Design review of the part built by this model. Coordinates are the model's own, in mm. A direction names the side the tool comes from. Give positions to 0.01 mm unless a question says otherwise; leave off trailing zeros. Order: outer loops, then holes, each group sorted by start corner. A loop starts at its lowest first (then second) coordinate and runs counter-clockwise, first axis right, second up. Notation, with made-up numbers: (3, -14) -> (7, -14) arc R19 cw to (7, -3) -> close; hole circle Ø3 at (36, 54.5). An arc over 180 degrees is marked (long way). Return JSON: item names as keys, results as strings.
```python
from build123d import *

# Parameters (mm, degrees)
F0_W     = 18.8512783498
F0_H     = 1.9018952735
F1_DEPTH = 1.016
F2_DEPTH = 0.3175
F4_DEPTH = 50.8


with BuildPart() as f1:
    # F0 (on Front) → F1 (new body, symmetric)
    with BuildSketch(Plane.XZ):
        with Locations((9.4256391749, -0.9509476367)):
            Rectangle(F0_W, F0_H)
    extrude(amount=F1_DEPTH, both=True)

    # F0 (on Front) → F2 (join, symmetric)
    with BuildSketch(Plane.XZ):
        with Locations((9.4256391749, -0.9509476367)):
            Rectangle(F0_W, F0_H)
        Polygon((18.8512783498, -1.9018952735), (0, -1.9018952735), (9.4256391749, -13.2702235132), align=None)
    extrude(amount=F2_DEPTH, both=True)

    # F3 (on face) → F4 (cut, symmetric)
    with BuildSketch(Plane.YZ.offset(18.8512783498)):
        Polygon((1.016, -1.9018952735), (1.016, 0), (0, -1.9018952735), (0.3175, -1.9018952735), align=None)
    extrude(amount=F4_DEPTH, both=True, mode=Mode.SUBTRACT)


solid = f1.part
```
Item 1: Add section B-B (y = -0.6). Give the boundary of the cut face in (x, z), plus the area to 3 significant figures.
Result set:
{"outline": "(0, -1.9) -> (18.85, -1.9) -> (18.85, 0) -> (0, 0) -> close", "area": "35.9 mm^2"}
Item 2: Machinability: for faces 1 (the face through (9, -0.318, -6)), 2 (the face through (0, 0, -1)), 3 (the face through (9, 0.318, -6)), which of the approach directions +Z, -Z, +X, -X, +Y, -Y give a long, thin tool a straight path to every point of the face, cutting with its end or side? Answer none if there is none.
Result set:
{"face 1": "-Z, +X, -X, -Y", "face 2": "+Z, -Z, -X, +Y, -Y", "face 3": "-Z, +X, -X, +Y"}
Item 3: Wall thickness on L1, parallel to Z at x = 10.25, y = -0.9; L2, parallel to Y at x = 2.5, z = -4.5; L3, parallel to Z at x = 1, y = 0.2: over which ranges is each line inside the solid? List them lowest first. Write a range as [from, to].
Result set:
{"L1": "z = [-1.9, 0]", "L2": "y = [-0.32, 0.32]", "L3": "z = [-3.11, -1.9], [-1.53, 0]"}
Item 4: Add section A-A (x = 15.75). Give the boundary of the cut face in (y, z).
Result set:
{"outline": "(-1.02, -1.9) -> (-0.32, -1.9) -> (-0.32, -5.64) -> (0.32, -5.64) -> (0.32, -1.9) -> (0, -1.9) -> (1.02, 0) -> (-1.02, 0) -> close"}
Item 5: Mouldability with a two-part tool opening along Z and no side actions: class faces 4 (the face through (14.07, 0, -7.67)), 5 (the face through (9.558, 0.515, -0.938)), 6 (the face through (9, -1.016, -1)) as released by +Z, released by -Z, zero draft, split by the parting line, or undercut.
Result set:
{"face 4": "released by -Z", "face 5": "undercut", "face 6": "zero draft"}
Item 6: Add section C-C (z = -2.5). Give the boundary of the cut face in (x, y), plus the area to 3 significant figures.
Result set:
{"outline": "(0.5, -0.32) -> (18.36, -0.32) -> (18.36, 0.32) -> (0.5, 0.32) -> close", "area": "11.3 mm^2"}
Item 7: Add section D-D (x = 8.75). Give the boundary of the cut face in (y, z), plus the area to 3 significant figures.
Result set:
{"outline": "(-1.02, -1.9) -> (-0.32, -1.9) -> (-0.32, -12.46) -> (0.32, -12.46) -> (0.32, -1.9) -> (0, -1.9) -> (1.02, 0) -> (-1.02, 0) -> close", "area": "9.60 mm^2"}
Item 8: For pin 1 (1 mm diameter, centred on x = 16.5, z = -4, fed in from -Y); pin 2 (1 mm diameter, centred on y = 0.5, z = -10, fed in from +X); pin 3 (1 mm diameter, centred on y = 0, z = -10.5, fed in from +X), all flat-tipped, find the tip position at first contact; note any pin that passes through.
Result set:
{"pin 1": "stops at y = -0.32", "pin 2": "stops at x = 12.52", "pin 3": "stops at x = 12.14"}
